For this review, take the finished solid that the model builds, in its own axes (mm). A direction names the side the tool comes from. Round coordinates to 2 decimals unless told otherwise and drop trailing zeros. Loops run counter-clockwise (first coordinate to the right, second up) from the corner with the lowest first, then second, coordinate; pieces in that order, holes last.
1. Tool access review of faces 5 (the cylindrical face through (22.269, -1.247, -5.616)), 6 (the cylindrical face through (12.789, -0.55, -2.477)): name each direction out of +Z, -Z, +X, -X, +Y, -Y from which nothing blocks a thin tool from reaching the whole face with its end or side.
2. Consider section C-C on x = 17.75. State the section outline as (y, z) points, then the cut area to 3 significant figures.
3. To check wall thickness, follow line 1 along Z through (x, y) = (21, 0); line 2 along Z through (x, y) = (4.25, 0); line 3 along X through (y, z) = (-3.25, 3.25). State the ranges of each line that lie inside material, in increasing order.
4. Consider section D-D on y = -3.5. State the section outline as (x, z) points, then the cut area to 3 significant figures.
5. Consider section A-A on z = 0. State the section outline as (x, y) points.
6. Clearance check with flat-ended pins moving along their axes: pin 1 Ø6 at (y, z) = (0.5, -2) entering from +X; pin 2 Ø4 at (x, y) = (6, 4) entering from +Z; pin 3 Ø3 at (y, z) = (0, 0) entering from +X; pin 4 Ø1.5 at (x, y) = (8.5, -4) entering from +Z. State where each tip first meets the part, or that it passes through.
7. Draft analysis for pull direction Y (two halves, no side actions). For faces 1 (the cylindrical face through (3.131, 0.385, 2.934)), 2 (the cylindrical face through (12.522, -8.187, 0.36)), 3 (the flat face through (19.05, 1.2, -2.5)), 4 (the flat face through (25.4, 2, 6)), state which applies: released by +Y, released by -Y, zero draft, split by the parting line, or undercut.
from build123d import *

# Parameters (mm, degrees)
F0_R     = 8.194552
F1_DEPTH = 25.4
F2_R     = 5.7531
F3_DEPTH = 6.35
F4_R     = 2.537622
F5_DEPTH = 19.051
F6_R     = 2.9591
F7_DEPTH = 6.35


with BuildPart() as f1:
    # F0 (on Right) → F1 (new body)
    with BuildSketch(Plane.YZ):
        Circle(F0_R)
    extrude(amount=F1_DEPTH)

    # F2 (on face) → F3 (cut)
    with BuildSketch(Plane.YZ.offset(25.4)):
        Circle(F2_R)
    extrude(amount=-F3_DEPTH, mode=Mode.SUBTRACT)

    # F4 (on face) → F5 (cut, through all)
    with BuildSketch(Plane.YZ.offset(19.05)):
        Circle(F4_R)
    extrude(amount=-F5_DEPTH, mode=Mode.SUBTRACT)

    # F6 (on face) → F7 (cut)
    with BuildSketch(Plane(origin=(0, 0, 0), x_dir=(0, -1, 0), z_dir=(-1, 0, 0))):
        Circle(F6_R)
    extrude(amount=-F7_DEPTH, mode=Mode.SUBTRACT)


solid = f1.part
Resolved:
1. face 5: +X
1. face 6: +X, -X
2. outline: circle Ø16.39 at (0, 0); hole circle Ø5.08 at (0, 0)
2. area: 191 mm2
3. line 1: z = -8.19 to -5.75, 5.75 to 8.19
3. line 2: z = -8.19 to -2.96, 2.96 to 8.19
3. line 3: x = 0 to 19.05
4. outline: (0, -7.41) - (25.4, -7.41) - (25.4, -4.57) - (19.05, -4.57) - (19.05, 4.57) - (25.4, 4.57) - (25.4, 7.41) - (0, 7.41) - close
4. area: 318 mm2
5. outline: (0, -8.19) - (25.4, -8.19) - (25.4, -5.75) - (19.05, -5.75) - (19.05, -2.54) - (6.35, -2.54) - (6.35, -2.96) - (0, -2.96) - close; (0, 2.96) - (6.35, 2.96) - (6.35, 2.54) - (19.05, 2.54) - (19.05, 5.75) - (25.4, 5.75) - (25.4, 8.19) - (0, 8.19) - close
6. pin 1: stops at x = 19.05
6. pin 2: stops at z = 7.95
6. pin 3: passes through
6. pin 4: stops at z = 7.52
7. face 1: undercut
7. face 2: split by the parting line
7. face 3: undercut
7. face 4: zero draft
